Check sheet for the modelled part. Datum: model origin and axes. Units: mm. Face numbers are marked on the shaded views. A direction names the side the tool comes from. Coordinates: 2 decimals unless noted, no trailing zeros. Order: outer loops, then holes, each group sorted by start corner. A loop starts at its lowest first (then second) coordinate and runs counter-clockwise, first axis right, second up.
1. Thickness scan on line 1 (X direction, y = -0.5, z = -3.5) (3 decimals); line 2 (Y direction, x = 12.7, z = -3) (3 decimals); line 3 (Y direction, x = -8, z = 11.5) (3 decimals). Record the ranges inside material, lowest first.
2. Set-up check for the marked faces 4 and 5: record each of +Z, -Z, +X, -X, +Y, -Y from which the full face is reachable in a straight line by a thin tool's end or side.
3. Draft check along X on the marked faces 1, 2 and 3. Enter one of: released by +X, released by -X, zero draft, split by the parting line, or undercut.
4. Cross-section at A-A (x = -12.7). Enter the section's corners in (y, z) (3 decimals).
5. Gauge pin test, flat ends, axial feed: pin 1 Ø0.8 at (x, y) = (-22.5, -17) entering from +Z; pin 2 Ø3 at (x, z) = (18, 13) entering from -Y (3 decimals); pin 3 Ø10 at (x, z) = (11.5, 12.5) entering from +Y. Record the tip position at first contact, or that the pin passes through.
6. Cross-section at C-C (z = 17.25). Enter the section's corners in (x, y) (3 decimals), then the cut area to 3 significant figures.
7. Cross-section at D-D (y = -9). Enter the section's corners in (x, z) (3 decimals).
8. Cross-section at B-B (y = 0). Enter the section's corners in (x, z) (3 decimals).
```python
from build123d import *

# Parameters (mm, degrees)
SKETCH1_W           = 57.15
SKETCH1_H           = 25.4
SKETCH1_R           = 8.382
BOSS_EXTRUDE1_DEPTH = 5.08
SKETCH3_W           = 25.4
SKETCH3_H           = 3.175
BOSS_EXTRUDE2_DEPTH = 57.15
SKETCH4_W           = 7.62
SKETCH4_H           = 4.572
CUT_EXTRUDE1_DEPTH  = 5.08
SKETCH5_W           = 5.08
SKETCH5_H           = 5.08
BOSS_EXTRUDE3_DEPTH = 2.54
CHAMFER1_SIZE       = 2.54


with BuildPart() as part:
    # Sketch1 → Boss-Extrude1 (new body)
    with BuildSketch(Plane.XY):
        Rectangle(SKETCH1_W, SKETCH1_H)
        with Locations((-12.7, 0)):
            Circle(SKETCH1_R, mode=Mode.SUBTRACT)
        with Locations((12.7, 0)):
            Circle(SKETCH1_R, mode=Mode.SUBTRACT)
    extrude(amount=-BOSS_EXTRUDE1_DEPTH)

    # Sketch3 → Boss-Extrude2 (add)
    with BuildSketch(Plane.ZY.offset(28.575)):
        with Locations((7.62, -14.2875)):
            Rectangle(SKETCH3_W, SKETCH3_H)
    extrude(amount=-BOSS_EXTRUDE2_DEPTH)

    # Sketch4 → Cut-Extrude1 (cut)
    with BuildSketch(Plane(origin=(0, -12.7, 0), x_dir=(1, 0, 0), z_dir=(0, 1, 0))):
        with Locations((-12.7, -7.62)):
            Rectangle(SKETCH4_W, SKETCH4_H)
        with Locations((12.7, -7.62)):
            Rectangle(SKETCH4_W, SKETCH4_H)
    extrude(amount=-CUT_EXTRUDE1_DEPTH, mode=Mode.SUBTRACT)

    # Sketch5 → Boss-Extrude3 (add)
    with BuildSketch(Plane.XZ.offset(15.875)):
        with Locations((-23.495, 7.62)):
            Rectangle(SKETCH5_W, SKETCH5_H)
        with Locations((23.495, 7.62)):
            Rectangle(SKETCH5_W, SKETCH5_H)
    extrude(amount=BOSS_EXTRUDE3_DEPTH)

    # Chamfer1
    chamfer1_edges = [part.edges().sort_by_distance(p)[0] for p in [
        (26.035, -18.415, 7.62),
        (-26.035, -18.415, 7.62),
    ]]
    chamfer(chamfer1_edges, length=CHAMFER1_SIZE - 0.0001)  # a hair under: the kernel refuses the full size


solid = part.part
```
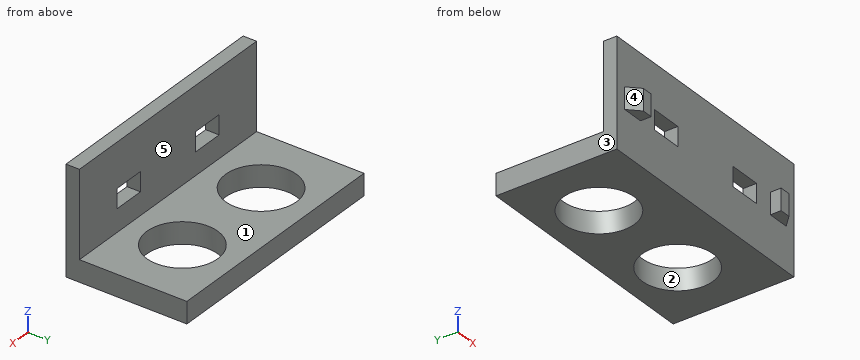
Data:
1. line 1: x = -28.575 to -21.067, -4.333 to 4.333, 21.067 to 28.575
1. line 2: y = -15.875 to -8.382, 8.382 to 12.7
1. line 3: y = -15.875 to -12.7
2. face 4: +Z, -Z, -X, -Y
2. face 5: +Z, +X, -X, +Y
3. face 1: zero draft
3. face 2: undercut
3. face 3: released by -X
4. outline: (-15.875, -5.08) - (-8.382, -5.08) - (-8.382, 0) - (-12.7, 0) - (-12.7, 5.334) - (-15.875, 5.334) - close; (-15.875, 9.906) - (-12.7, 9.906) - (-12.7, 20.32) - (-15.875, 20.32) - close; (8.382, -5.08) - (12.7, -5.08) - (12.7, 0) - (8.382, 0) - close
5. pin 1: stops at z = 10.16
5. pin 2: stops at y = -15.875
5. pin 3: stops at y = -12.7
6. outline: (-28.575, -15.875) - (28.575, -15.875) - (28.575, -12.7) - (-28.575, -12.7) - close
6. area: 181 mm2
7. outline: (-28.575, -5.08) - (28.575, -5.08) - (28.575, 0) - (-28.575, 0) - close
8. outline: (-28.575, -5.08) - (-21.082, -5.08) - (-21.082, 0) - (-28.575, 0) - close; (-4.318, -5.08) - (4.318, -5.08) - (4.318, 0) - (-4.318, 0) - close; (21.082, -5.08) - (28.575, -5.08) - (28.575, 0) - (21.082, 0) - close
